from build123d import *

# Parameters (mm, degrees)
F1_DEPTH  = 18.1
F3_DEPTH  = 2.5
F4_W      = 55
F4_H      = 17
F5_DEPTH  = 1
F6_R      = 0.5
F7_W      = 16.7
F7_H      = 18.3
F8_DEPTH  = 5.5
F9_R      = 0.5
F10_W     = 6
F10_H     = 3
F11_DEPTH = 10
F12_R     = 1.5
F13_DEPTH = 5


with BuildPart() as f1:
    # F0 (on Top) → F1 (new body)
    with BuildSketch(Plane.XY):
        Polygon((69.9801715439, -2.5), (35.05, 0), (0.1198284561, -2.5), (4.6301715439, -96.6), (35.05, -99.1), (65.4698284561, -96.6), align=None)
    extrude(amount=F1_DEPTH)

    # F2 (on face) → F3 (join)
    with BuildSketch(Plane.XY.offset(18.1)):
        with BuildLine():
            Line((25.1822125728, -66.8218548894), (44.778130515, -66.8218548894))
            ThreePointArc((44.778130515, -66.8218548894), (34.9801715439, -58.8218548894), (25.1822125728, -66.8218548894))
        make_face()
        with BuildLine():
            ThreePointArc((25.1822125728, -70.8218548894), (34.9801715439, -78.8218548894), (44.778130515, -70.8218548894))
            Line((44.778130515, -70.8218548894), (25.1822125728, -70.8218548894))
        make_face()
    extrude(amount=F3_DEPTH)

    # F4 (on face) → F5 (cut)
    with BuildSketch(Plane.XY.offset(18.1)):
        with Locations((35.05, -29.5)):
            Rectangle(F4_W, F4_H)
    extrude(amount=-F5_DEPTH, mode=Mode.SUBTRACT)

    # F6
    f6_edges = [f1.edges().sort_by_distance(p)[0] for p in [
        (34.980172, -66.821855, 20.6),
        (34.980172, -58.821855, 20.6),
        (34.980172, -78.821855, 20.6),
        (34.980172, -70.821855, 20.6),
        (25.182213, -70.821855, 19.35),
        (44.778131, -66.821855, 19.35),
        (25.182213, -66.821855, 19.35),
        (44.778131, -70.821855, 19.35),
        (65.469828, -96.6, 9.05),
        (69.980172, -2.5, 9.05),
        (67.725, -49.55, 0),
        (67.725, -49.55, 18.1),
        (35.05, -99.1, 9.05),
        (50.259914, -97.85, 0),
        (50.259914, -97.85, 18.1),
        (4.630172, -96.6, 9.05),
        (19.840086, -97.85, 0),
        (19.840086, -97.85, 18.1),
        (0.119828, -2.5, 9.05),
        (2.375, -49.55, 0),
        (2.375, -49.55, 18.1),
        (35.05, 0, 9.05),
        (17.584914, -1.25, 0),
        (17.584914, -1.25, 18.1),
        (52.515086, -1.25, 0),
        (52.515086, -1.25, 18.1),
    ]]
    fillet(f6_edges, radius=F6_R)

    # F7 (on face) → F8 (join)
    with BuildSketch(Plane(origin=(0, 0, 0), x_dir=(1, 0, 0), z_dir=(0, 0, -1))):
        with Locations((35.0856943769, 28.15)):
            Rectangle(F7_W, F7_H)
    extrude(amount=F8_DEPTH)

    # F9
    f9_edges = [f1.edges().sort_by_distance(p)[0] for p in [
        (35.085694, -37.3, -5.5),
        (26.735694, -28.15, -5.5),
        (35.085694, -19, -5.5),
        (43.435694, -28.15, -5.5),
        (43.435694, -19, -2.75),
        (26.735694, -19, -2.75),
        (26.735694, -37.3, -2.75),
        (43.435694, -37.3, -2.75),
    ]]
    fillet(f9_edges, radius=F9_R)

    # F10 (on face) → F11 (cut)
    with BuildSketch(Plane(origin=(0, 0, -5.5), x_dir=(1, 0, 0), z_dir=(0, 0, -1))):
        Polygon((38.0856943769, 26), (41.4356943769, 26), (41.4356943769, 33), (28.7356943769, 33), (28.7356943769, 26), (32.0856943769, 26), align=None)
        with Locations((35.0856943769, 24.5)):
            Rectangle(F10_W, F10_H)
    extrude(amount=-F11_DEPTH, mode=Mode.SUBTRACT)

    # F12 (on face) → F13 (cut)
    with BuildSketch(Plane(origin=(0, 0, 0), x_dir=(1, 0, 0), z_dir=(0, 0, -1))):
        with Locations((4.5356943769, 7)):
            Circle(F12_R)
        with Locations((60.4856943769, 93.6)):
            Circle(F12_R)
    extrude(amount=-F13_DEPTH, mode=Mode.SUBTRACT)


solid = f1.part
Could you check a few things on this model? Use its own coordinates, in mm. A direction names the side the tool comes from. Give positions to 0.01 mm unless a question says otherwise; leave off trailing zeros. Order: outer loops, then holes, each group sorted by start corner. A loop starts at its lowest first (then second) coordinate and runs counter-clockwise, first axis right, second up. Notation, with made-up numbers: (-30, 43) -> (29, 43) arc R22 ccw to (29, 69) -> close; hole circle Ø5 at (-14.75, -29.75). An arc over 180 degrees is marked (long way). Answer in a Markdown table with one row per item. Add a question column.
Item 1: We'd pull the mould along Y, two halves only. Please class faces 4 (the cylindrical face through (50.259, -97.699, 0.143)), 5 (the flat face through (40, -26, -1)), 6 (the flat face through (43.436, -28, -2)): pulls with the +Y half, pulls with the -Y half, needs draft (parallel to the pull), parting line crosses it, or undercut.
Item 2: Please list where these lines run through material, in increasing order: probe 1 along Z at (x, y) = (40.5, -75); probe 2 along X at (y, z) = (-93.6, 2.05); probe 3 along Z at (x, y) = (60, -29.5).
Item 3: For faces 1 (the flat face through (41.436, -29, -1)), 2 (the flat face through (26.736, -28, -2)), 3 (the flat face through (35, -19, -2)), which set-ups out of +Z, -Z, +X, -X, +Y, -Y let a thin tool reach every point of the face, with its end or its side?
Item 4: Imagine slicing it at A-A (z = 3.5). List the corners of the cut face in (x, y) for me, and give its area (3 significant figures).
Item 5: Imagine slicing it at B-B (z = 15). List the corners of the cut face in (x, y) for me, and give its area (3 significant figures).
Item 6: I'm going to push flat-ended pins straight in: P1, Ø3.5, axis at y = -30.5, z = -1, coming from the +X side; P2, Ø1.5, axis at y = -26.5, z = -3, coming from the +X side; P3, Ø3, axis at x = 25, z = 9, coming from the -Y side. Where does each tip first touch, or does it pass through?
Result:
| question | item | result |
|---|---|---|
| 1 | face 4 | pulls with the -Y half |
| 1 | face 5 | undercut |
| 1 | face 6 | needs draft |
| 2 | probe 1 | 0 to 20.6 |
| 2 | probe 2 | 4.49 to 58.99, 61.99 to 65.61 |
| 2 | probe 3 | 0 to 17.1 |
| 3 | face 1 | -Z |
| 3 | face 2 | -Z, -X, +Y, -Y |
| 3 | face 3 | -Z, +X, -X, +Y |
| 4 | outline | (0.14, -2.99) -> (4.61, -96.16) arc R0.5 ccw to (5.07, -96.64) -> (35.01, -99.1) arc R0.5 ccw to (35.09, -99.1) -> (65.03, -96.64) arc R0.5 ccw to (65.49, -96.16) -> (69.96, -2.99) arc R0.5 ccw to (69.49, -2.47) -> (35.09, 0) arc R0.5 ccw to (35.01, 0) -> (0.61, -2.47) arc R0.5 ccw to start; hole circle Ø3 at (4.54, -7); hole (28.74, -33) -> (41.44, -33) -> (41.44, -26) -> (38.09, -26) -> (38.09, -23) -> (32.09, -23) -> (32.09, -26) -> (28.74, -26) -> close; hole circle Ø3 at (60.49, -93.6) |
| 4 | area | 6,190 mm2 |
| 5 | outline | (0.14, -2.99) -> (4.61, -96.16) arc R0.5 ccw to (5.07, -96.64) -> (35.01, -99.1) arc R0.5 ccw to (35.09, -99.1) -> (65.03, -96.64) arc R0.5 ccw to (65.49, -96.16) -> (69.96, -2.99) arc R0.5 ccw to (69.49, -2.47) -> (35.09, 0) arc R0.5 ccw to (35.01, 0) -> (0.61, -2.47) arc R0.5 ccw to start |
| 5 | area | 6,310 mm2 |
| 6 | P1 | x = 68.68 |
| 6 | P2 | x = 43.44 |
| 6 | P3 | y = -98.4 |
